Design review of the part built by this model. Coordinates are the model's own, in mm. A direction names the side the tool comes from. Give positions to 0.01 mm unless a question says otherwise; leave off trailing zeros. Order: outer loops, then holes, each group sorted by start corner. A loop starts at its lowest first (then second) coordinate and runs counter-clockwise, first axis right, second up. Notation, with made-up numbers: (79.5, -17) -> (134.5, -17) arc R15 ccw to (134.5, -5) -> close; hole circle Ø1 at (55.25, -10). An arc over 180 degrees is marked (long way). Return JSON: item names as keys, results as strings.
```python
from build123d import *

# Parameters (mm, degrees)
SKETCH1_R           = 1.524
SKETCH1_R_2         = 3.175
SKETCH1_R_3         = 2.667
SKETCH1_R_4         = 34.04
BOSS_EXTRUDE1_DEPTH = 4.7625
SKETCH2_R           = 1.1303
CUT_EXTRUDE1_DEPTH  = 6.35


with BuildPart() as part:
    # Sketch1 → Boss-Extrude1 (new body)
    with BuildSketch(Plane(origin=(0, 0, 0), x_dir=(0, 0, -1), z_dir=(1, 0, 0))):
        with BuildLine():
            Line((-28.170295117, 0), (77.382795117, 0))
            ThreePointArc((77.382795117, 0), (79.627859148, 0.92993597), (80.557795117, 3.175))
            Line((80.557795117, 3.175), (80.557795117, 40.132))
            ThreePointArc((80.557795117, 40.132), (80.175158576, 42.302961389), (79.073362565, 44.212288398))
            add(Edge.make_bspline(
                [(-34.867281509, 119.579027078), (-0.058341562, 112.208593965), (41.263784204, 89.298575374), (79.073362565, 44.212288398)],
                knots=[0, 0, 0, 0, 1, 1, 1, 1], degree=3))
            ThreePointArc((-34.867281509, 119.579027078), (-66.539067219, 111.95566221), (-80.557795117, 82.55))
            Line((-80.557795117, 82.55), (-80.557795117, 50.292))
            Line((-80.557795117, 50.292), (-75.795295117, 50.292))
            Line((-75.795295117, 50.292), (-75.795295117, 40.132))
            Line((-75.795295117, 40.132), (-31.345295117, 40.132))
            Line((-31.345295117, 40.132), (-31.345295117, 3.175))
            ThreePointArc((-31.345295117, 3.175), (-30.415359148, 0.92993597), (-28.170295117, 0))
        make_face()
        with Locations(Location((-78.176545117, 55.372, 0), (0, 0, 180))):
            Circle(SKETCH1_R, mode=Mode.SUBTRACT)
        with Locations(Location((1.992204883, 100.457, 0), (0, 0, 180))):
            Circle(SKETCH1_R_2, mode=Mode.SUBTRACT)
        with Locations(Location((-14.692204883, 20.066, 0), (0, 0, 180))):
            Circle(SKETCH1_R_3, mode=Mode.SUBTRACT)
        with Locations(Location((-42.707795117, 82.55, 0), (0, 0, 180))):
            Circle(SKETCH1_R_4, mode=Mode.SUBTRACT)
        with BuildLine():
            Line((67.857795117, 15.3035), (57.697795117, 15.3035))
            ThreePointArc((57.697795117, 15.3035), (52.935295117, 20.066), (57.697795117, 24.8285))
            Line((57.697795117, 24.8285), (67.857795117, 24.8285))
            ThreePointArc((67.857795117, 24.8285), (72.620295117, 20.066), (67.857795117, 15.3035))
        make_face(mode=Mode.SUBTRACT)
    extrude(amount=BOSS_EXTRUDE1_DEPTH)

    # Sketch2 → Cut-Extrude1 (cut)
    with BuildSketch(Plane.XY.offset(75.795295117)):
        with Locations((2.38125, 45.212)):
            Circle(SKETCH2_R)
    extrude(amount=-CUT_EXTRUDE1_DEPTH, mode=Mode.SUBTRACT)


solid = part.part
```
Item 1: Wall thickness on L1, parallel to Y at x = 4.55, z = 46.5; L2, parallel to Y at x = 0.5, z = 25; L3, parallel to Z at x = 3.3, y = 32: over which ranges is each line inside the solid? List them lowest first. Write a range as [from, to].
Result set:
{"L1": "y = [40.13, 48.72], [116.38, 120.21]", "L2": "y = [0, 53.48], [111.62, 117.12]", "L3": "z = [-80.56, 31.35]"}
Item 2: Mouldability with a two-part tool opening along Z and no side actions: class faces 1 (the face through (2, 40.132, 54)), 2 (the face through (2, 21, -80.558)), 3 (the face through (2, 15.304, -63)) as released by +Z, released by -Z, zero draft, split by the parting line, or undercut.
Result set:
{"face 1": "zero draft", "face 2": "released by -Z", "face 3": "undercut"}
Item 3: Machinability: for faces 4 (the face through (2.9, 46.4, 75.795)), 5 (the face through (2.3, 0.9, -79.6)), 6 (the face through (2, 24.828, -63)), which of the approach directions +Z, -Z, +X, -X, +Y, -Y give a long, thin tool a straight path to every point of the face, cutting with its end or side? Answer none if there is none.
Result set:
{"face 4": "+Z, +X, -X, -Y", "face 5": "-Z, +X, -X, -Y", "face 6": "+X, -X"}
Item 4: Add section A-A (y = 9.5). Give the boundary of the cut face in (x, z).
Result set:
{"outline": "(0, -80.56) -> (4.76, -80.56) -> (4.76, 31.35) -> (0, 31.35) -> close"}
Item 5: Add section B-B (x = 2.3). Give the number of separate pieces and of enclosed holes in the cut face, plus the area to 3 significant figures.
Result set:
{"separate pieces": "1", "enclosed holes": "5", "area": "9,700 mm^2"}
Item 6: For pin 1 (2 mm diameter, centred on y = 28.5, z = 4.5, fed in from -X); pin 2 (2 mm diameter, centred on x = 2.38, y = 45.21, fed in from +Z); pin 3 (1.4 mm diameter, centred on x = 2.5, y = 25, fed in from +Z); pin 4 (1.4 mm diameter, centred on x = 3, z = 58, fed in from -Y), all flat-tipped, find the tip position at first contact; note any pin that passes through.
Result set:
{"pin 1": "stops at x = 0", "pin 2": "stops at z = 69.45", "pin 3": "stops at z = 31.35", "pin 4": "stops at y = 40.13"}
